from build123d import *

# Parameters (mm, degrees)
F0_W     = 804
F0_H     = 800
F0_H_2   = 285
F1_DEPTH = 490
F2_W     = 100
F2_H     = 2180
F3_DEPTH = 18


with BuildPart() as f1:
    # F0 (on Front) → F1 (new body)
    with BuildSketch(Plane.XZ):
        Polygon((0, 2180), (0, 0), (18, 0), (18, 720), (822, 720), (822, 0), (840, 0), (840, 2180), (822, 2180), (822, 2162), (822, 1877), (18, 1877), (18, 2162), (18, 2180), align=None)
        with Locations((420, 1156)):
            Rectangle(F0_W, F0_H, mode=Mode.SUBTRACT)
        with Locations((420, 1716.5)):
            Rectangle(F0_W, F0_H_2, mode=Mode.SUBTRACT)
    extrude(amount=F1_DEPTH)

    # F2 (on face) → F3 (join)
    with BuildSketch(Plane.YZ.offset(840)):
        with Locations((-540, 1090)):
            Rectangle(F2_W, F2_H)
    extrude(amount=-F3_DEPTH)


solid = f1.part
Read the model definition and answer for the solid it produces. Units are mm, in the model's axes. A direction names the side the tool comes from. Coordinates: 2 decimals unless noted, no trailing zeros. Order: outer loops, then holes, each group sorted by start corner. A loop starts at its lowest first (then second) coordinate and runs counter-clockwise, first axis right, second up. Notation, with made-up numbers: (87.5, 66.25) - (128.5, 66.25) arc R8 cw to (128.5, 73.25) - close; hole circle Ø7 at (0.5, 30.5). An arc over 180 degrees is marked (long way). Use one line per item in the form item = value.
(1) Section C-C, the plane y = -163.5 is taken. Give the vertices of the cut face in (x, z), then the cut area to 3 significant figures.
Computed values:
outline = (0, 0) - (18, 0) - (18, 720) - (822, 720) - (822, 0) - (840, 0) - (840, 2180) - (822, 2180) - (822, 1877) - (18, 1877) - (18, 2180) - (0, 2180) - close; hole (18, 756) - (822, 756) - (822, 1556) - (18, 1556) - close; hole (18, 1574) - (822, 1574) - (822, 1859) - (18, 1859) - close
area = 136,000 mm²
(2) Given pin 1 Ø3 at (x, y) = (118, -416.5) entering from +Z, flat-ended and moving along its own axis, determine where the tip first touches the part or whether it passes through.
Computed values:
pin_1 = 1877
(3) Section A-A, the plane z = 1065 is taken. Give the vertices of the cut face in (x, y), then the cut area to 3 significant figures.
Computed values:
outline = (0, -490) - (18, -490) - (18, 0) - (0, 0) - close; (822, -590) - (840, -590) - (840, 0) - (822, 0) - close
area = 19,400 mm²
(4) For a pull along Z with two mould halves and no side action, classify faces 5 (the face through (414, -242, 756)), 6 (the face through (18, -242, 2026)), 7 (the face through (426, -242, 1877)) as pulls with the +Z half, pulls with the -Z half, needs draft (parallel to the pull), parting line crosses it, or undercut.
Computed values:
face_5 = undercut
face_6 = needs draft
face_7 = pulls with the +Z half
(5) Which of the six approach directions +Z, -Z, +X, -X, +Y, -Y give full straight-line access (tool end or side, diameter ignored) to faces 1 (the face through (18, -242, 355)), 2 (the face through (414, -242, 1859)), 3 (the face through (13, -490, 1095)), 4 (the face through (822.5, 0, 1095.1))?
Computed values:
face_1 = -Z, +Y, -Y
face_2 = +Y, -Y
face_3 = +Z, -Z, -X, -Y
face_4 = +Z, -Z, +X, -X, +Y
(6) Section B-B, the plane x = 318.5 is taken. Give the vertices of the cut face in (y, z), then the cut area to 3 significant figures.
Computed values:
outline = (-490, 720) - (0, 720) - (0, 756) - (-490, 756) - close; (-490, 1556) - (0, 1556) - (0, 1574) - (-490, 1574) - close; (-490, 1859) - (0, 1859) - (0, 1877) - (-490, 1877) - close
area = 35,300 mm²
(7) Straight lines are drawn through the part: L1, parallel to Z at x = 554.5, y = -306.5; L2, parallel to X at y = -485.5, z = 239; L3, parallel to X at y = -496, z = 340.5. For each, find the intervals that lie inside material, in ascending order.
Computed values:
L1 = 720 to 756, 1556 to 1574, 1859 to 1877
L2 = 0 to 18, 822 to 840
L3 = 822 to 840
